```python
from build123d import *

# Parameters (mm, degrees)
REVOLVE2_ANGLE = 180
FILLET1_R      = 2
FILLET2_R      = 2


with BuildPart() as part:
    # Sketch1 → Revolve2 (revolve)
    with BuildSketch(Plane.XY):
        Polygon((298.984408478, 58.041083961), (302.019314835, 58.041083961), (304.061664281, 44.775692844), (308.932649078, 44.775692844), (311.24430288, 38.005849568), (313.986310635, 38.005849568), (313.986310635, 38.974632238), (312.008767265, 38.974632238), (309.907518568, 45.829224513), (308.932649078, 45.829224513), (305.095386851, 45.829224513), (302.974041332, 58.990397452), (300.078054647, 58.990397452), (300.078054647, 66.023507974), (298.984408478, 66.023507974), align=None)
    revolve(axis=Axis((321.047285869, 38.005849568, 0), (0, 1, 0)), revolution_arc=REVOLVE2_ANGLE)

    # Fillet1
    fillet1_edges = [part.edges().sort_by_distance(p)[0] for p in [
        (321.047285869, 58.041083961, 22.062877391),
    ]]
    fillet(fillet1_edges, radius=FILLET1_R)

    # Fillet2
    fillet2_edges = [part.edges().sort_by_distance(p)[0] for p in [
        (321.047285869, 44.775692844, 16.985621588),
    ]]
    fillet(fillet2_edges, radius=FILLET2_R)


solid = part.part
```
Verification items for the finished model (mm, model axes). A direction names the side the tool comes from. Round coordinates to 2 decimals unless told otherwise and drop trailing zeros. Write each loop counter-clockwise with the first axis right and the second up, starting at its lowest first coordinate (ties: lowest second). Pieces come first, ordered by that corner, then holes.
1. Access from +Z, -Z, +X, -X, +Y, -Y to the whole of each face (thin tool, end or side, straight path). Record for faces 1 (the flat face through (321, 45.829, 12)), 2 (the cylindrical face through (320.562, 62.99, 22.058)), 3 (the flat face through (318, 58.041, 19)).
2. Scan lines: L1, parallel to X at y = 57.5, z = 3.5; L2, parallel to X at y = 43.75, z = 4.75; L3, parallel to Y at x = 309, z = 9. Record each from-to range of solid material in increasing order.
3. Gauge pin test, flat ends, axial feed: P1, Ø1, axis at y = 58, z = 7, coming from the -X side; P2, Ø10, axis at y = 52.5, z = 9.5, coming from the -X side; P3, Ø5, axis at y = 41.5, z = 9.5, coming from the -X side; P4, Ø4, axis at x = 312, z = 7, coming from the -Y side. Record the tip position at first contact, or that the pin passes through.
4. Section check B-B on y = 44. Enter the section's corners in (x, z).
5. Draft check along X on faces 4 (the conical face through (320.83, 41.69, 9.87)), 5 (the conical face through (320.818, 39.839, 10.426)), 6 (the cylindrical face through (320.586, 62.556, 20.964)), 7 (the flat face through (321, 44.776, 13)). Enter one of: +X half, -X half, draft (parallel to the pull), parting line (faces both ways), or undercut.
Answer:
1. face 1: -Z, +Y
1. face 2: +Z, +Y, -Y
1. face 3: +Z, -Y
2. L1: x = 302.43 to 303.56, 338.53 to 339.67
2. L2: x = 310.28 to 311.68, 330.41 to 331.81
2. L3: y = 44.78 to 45.83
3. P1: stops at x = 300.87
3. P2: stops at x = 303.22
3. P3: stops at x = 312.29
3. P4: stops at y = 38.01
4. outline: (309.2, 0) - (310.47, 0) arc R10.58 cw to (331.63, 0) - (332.9, 0) arc R11.85 ccw to start
5. face 4: undercut
5. face 5: parting line
5. face 6: undercut
5. face 7: draft
